```python
from build123d import *

# Parameters (mm, degrees)
F0_R     = 2.25
F0_R_2   = 16
F1_DEPTH = 1


with BuildPart() as f1:
    # F0 (on Front) → F1 (new body)
    with BuildSketch(Plane.XZ):
        with BuildLine():
            Line((4.209625, -2.647812), (4.209625, 1.420013))
            ThreePointArc((4.209625, 1.420013), (15.207091, 0.758549), (25.341338, 5.080448))
            Line((25.341338, 5.080448), (27.98607, 2.162959))
            ThreePointArc((27.98607, 2.162959), (33.227056, 2.037489), (33.08977, 7.27818))
            Line((33.08977, 7.27818), (30.211789, 9.875299))
            ThreePointArc((30.211789, 9.875299), (27.548758, 41.893357), (-4.572665, 42.57308))
            Line((-4.572665, 42.57308), (-8.227887, 46.289463))
            ThreePointArc((-8.227887, 46.289463), (-13.224062, 46.363974), (-13.364673, 41.369222))
            Line((-13.364673, 41.369222), (-11.350405, 39.209819))
            ThreePointArc((-11.350405, 39.209819), (-14.650167, 33.0315), (-15.790375, 26.12064))
            Line((-15.790375, 26.12064), (-15.790375, -2.647812))
            Line((-15.790375, -2.647812), (4.209625, -2.647812))
        make_face()
        with Locations((30.666229, 4.592549)):
            Circle(F0_R, mode=Mode.SUBTRACT)
        with Locations((12.784705, 22.352362)):
            Circle(F0_R_2, mode=Mode.SUBTRACT)
        with Locations((-10.763726, 43.795356)):
            Circle(F0_R, mode=Mode.SUBTRACT)
    extrude(amount=F1_DEPTH)


solid = f1.part
```
Geometry check sheet. Reference: the model listing, model coordinates, mm. A direction names the side the tool comes from. Give positions to 0.01 mm unless a question says otherwise; leave off trailing zeros. Order: outer loops, then holes, each group sorted by start corner. A loop starts at its lowest first (then second) coordinate and runs counter-clockwise, first axis right, second up. Notation, with made-up numbers: (61.5, -35) -> (118.5, -35) arc R29 cw to (118.5, -14) -> close; hole circle Ø2 at (13, -5). An arc over 180 degrees is marked (long way). Write each question's results on one line, items separated by ' | '. Start each with the question number.
(1) Sectioned sample at D-D (y = -0.75). Enter the section's corners in (x, z).
(2) Sectioned sample at A-A (z = 8). Enter the section's corners in (x, y), plus the area to 3 significant figures.
(3) Sectioned sample at C-C (x = 8.5). Enter the section's corners in (y, z).
(4) Mould release check, pull along X, two halves, no side actions. Record for faces 4 (the face through (-12.37, -0.49, 40.3)), 5 (the face through (31.67, -0.49, 8.56)), 6 (the face through (21.39, -0.49, 35.84)): pulls with the +X half, pulls with the -X half, needs draft (parallel to the pull), parting line crosses it, or undercut.
(5) Scan lines: line 1 (Z direction, x = 6.5, y = -0.1); line 2 (X direction, y = -0.2, z = 28.5); line 3 (Z direction, x = 25.5, y = -0.2). Record each from-to range of solid material in increasing order.
(6) Sectioned sample at B-B (x = 32). Enter the section's corners in (y, z), plus the area to 3 significant figures.
(7) Access from +Z, -Z, +X, -X, +Y, -Y to the whole of each face (thin tool, end or side, straight path). Record for faces 1 (the face through (-6.375, -0.493, 44.405)), 2 (the face through (26.645, -0.493, 3.642)), 3 (the face through (-14.62, -0.49, 33.12)).
Answer below:
1) outline: (-15.79, -2.65) -> (4.21, -2.65) -> (4.21, 1.42) arc R24 ccw to (25.34, 5.08) -> (27.99, 2.16) arc R3.62 ccw (long way) to (33.09, 7.28) -> (30.21, 9.88) arc R24 ccw to (-4.57, 42.57) -> (-8.23, 46.29) arc R3.56 ccw to (-13.36, 41.37) -> (-11.35, 39.21) arc R21.51 ccw to (-15.79, 26.12) -> close; hole circle Ø4.5 at (-10.76, 43.8); hole circle Ø32 at (12.78, 22.35); hole circle Ø4.5 at (30.67, 4.59)
2) outline: (-15.79, -1) -> (5.71, -1) -> (5.71, 0) -> (-15.79, 0) -> close; (19.86, -1) -> (32.29, -1) -> (32.29, 0) -> (19.86, 0) -> close | area: 33.9 mm2
3) outline: (-1, 0.55) -> (0, 0.55) -> (0, 6.94) -> (-1, 6.94) -> close; (-1, 37.77) -> (0, 37.77) -> (0, 48.26) -> (-1, 48.26) -> close
4) face 4: pulls with the -X half | face 5: pulls with the +X half | face 6: undercut
5) line 1: 0.85 to 7.64, 37.07 to 47.96 | line 2: -15.66 to -1.99, 27.56 to 34.76 | line 3: 4.91 to 12.64, 32.06 to 43.61
6) outline: (-1, 1.23) -> (0, 1.23) -> (0, 2.78) -> (-1, 2.78) -> close; (-1, 6.4) -> (0, 6.4) -> (0, 8.26) -> (-1, 8.26) -> close; (-1, 12.59) -> (0, 12.59) -> (0, 36.22) -> (-1, 36.22) -> close | area: 27.0 mm2
7) face 1: +Z, +Y, -Y | face 2: -Z, +Y, -Y | face 3: -X, +Y, -Y
